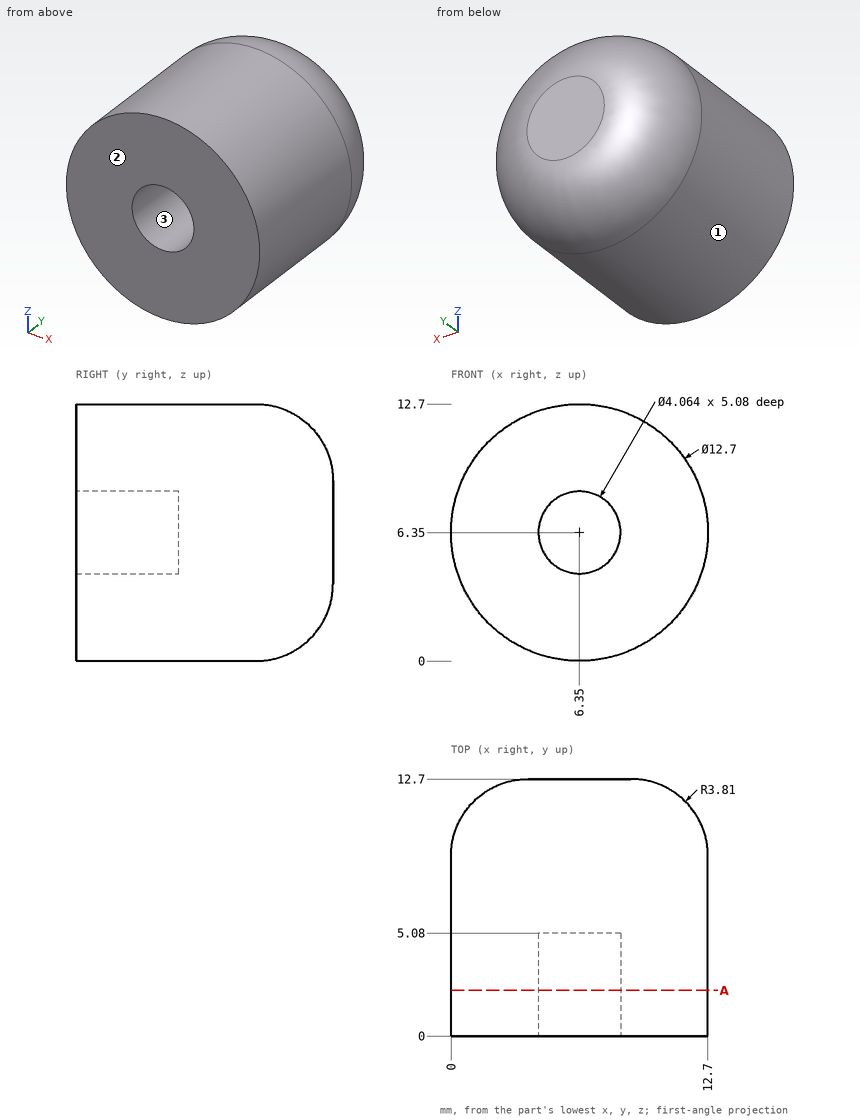
Geometry check sheet. Reference: drawing and pictorial views, mm from the part's lowest x, y, z. Round coordinates to 2 decimals unless told otherwise and drop trailing zeros. Write each loop counter-clockwise with the first axis right and the second up, starting at its lowest first coordinate (ties: lowest second). Pieces come first, ordered by that corner, then holes.
1. Draft check along Z on the marked faces 1, 2 and 3. Enter one of: +Z half, -Z half, draft (parallel to the pull), parting line (faces both ways), or undercut.
2. Scan lines: L1, parallel to X at y = 3.9, z = 6.35; L2, parallel to Z at x = 5.25, y = 3.75. Record each from-to range of solid material in increasing order.
3. Gauge pin test, flat ends, axial feed: P1, Ø1.5, axis at y = 11.5, z = 4.5, coming from the -X side; P2, Ø1, axis at y = 4, z = 5.5, coming from the -X side; P3, Ø2, axis at x = 6, y = 5.5, coming from the -Z side; P4, Ø1.2, axis at x = 5.5, z = 5.5, coming from the -Y side. Record the tip position at first contact, or that the pin passes through.
4. Section check A-A on y = 2.25. Enter the section's corners in (x, z).
Answer:
1. face 1: parting line
1. face 2: draft
1. face 3: undercut
2. L1: x = 0 to 4.32, 8.38 to 12.7
2. L2: z = 0.1 to 4.64, 8.06 to 12.6
3. P1: stops at x = 0.73
3. P2: stops at x = 0.01
3. P3: stops at z = 0
3. P4: stops at y = 5.08
4. outline: circle Ø12.7 at (6.35, 6.35); hole circle Ø4.06 at (6.35, 6.35)
